CAD build for the part. Positions are in the model's coordinates, mm. A direction names the side the tool comes from. Round coordinates to 2 decimals unless told otherwise and drop trailing zeros. Order: outer loops, then holes, each group sorted by start corner. A loop starts at its lowest first (then second) coordinate and runs counter-clockwise, first axis right, second up. Notation, with made-up numbers: M 14,58.5 L 40,58.5 A28 cw 40,97.5 Z; hole C 40.25,-35 d1. An arc over 180 degrees is marked long. Answer as CSV lines item,"result". Start each with the question number.
```python
from build123d import *

# Parameters (mm, degrees)
SKETCH2_W           = 15
SKETCH2_H           = 15
SKETCH2_W_2         = 30
SKETCH2_R           = 4.15
BOSS_EXTRUDE1_DEPTH = 10
SKETCH2_3_W         = 15
SKETCH2_3_H         = 15
SKETCH2_3_W_2       = 30
SKETCH2_3_R         = 4.15
BOSS_EXTRUDE2_DEPTH = 10
SKETCH4_R           = 1.6
CUT_EXTRUDE1_DEPTH  = 36
CUT_EXTRUDE2_START  = -6.25
SKETCH4_3_R         = 1.6
CUT_EXTRUDE2_DEPTH  = 2.5
SKETCH5_W           = 45
SKETCH5_H           = 5
BOSS_EXTRUDE3_DEPTH = 75
SKETCH6_W           = 45
SKETCH6_H           = 5
BOSS_EXTRUDE4_DEPTH = 15
SKETCH7_W           = 5
SKETCH7_H           = 20
BOSS_EXTRUDE5_DEPTH = 45
CUT_EXTRUDE3_REACH  = 119.58
SKETCH8_R           = 1.6
CUT_EXTRUDE4_START  = -1.25
CUT_EXTRUDE4_DEPTH  = 2.5


with BuildPart() as part:
    # Sketch2 → Boss-Extrude1 (new body)
    with BuildSketch(Plane(origin=(0, 0, 0), x_dir=(1, 0, 0), z_dir=(0, 1, 0))):
        with Locations((22.5, 0)):
            Rectangle(SKETCH2_W, SKETCH2_H)
        Rectangle(SKETCH2_W_2, SKETCH2_H)
        with Locations(Location((7.5, 0, 0), (0, 0, 270))):
            Circle(SKETCH2_R, mode=Mode.SUBTRACT)
        with Locations(Location((-7.5, 0, 0), (0, 0, 270))):
            Circle(SKETCH2_R, mode=Mode.SUBTRACT)
    extrude(amount=BOSS_EXTRUDE1_DEPTH)

    # Sketch2_3 → Boss-Extrude2 (add)
    with BuildSketch(Plane(origin=(0, 0, 0), x_dir=(1, 0, 0), z_dir=(0, 1, 0))):
        with Locations((22.5, 0)):
            Rectangle(SKETCH2_3_W, SKETCH2_3_H)
        Rectangle(SKETCH2_3_W_2, SKETCH2_3_H)
        with Locations(Location((7.5, 0, 0), (0, 0, 270))):
            Circle(SKETCH2_3_R, mode=Mode.SUBTRACT)
        with Locations(Location((-7.5, 0, 0), (0, 0, 270))):
            Circle(SKETCH2_3_R, mode=Mode.SUBTRACT)
        with Locations(Location((-7.5, 0, 0), (0, 0, 270))):
            Circle(SKETCH2_3_R)
        with Locations(Location((7.5, 0, 0), (0, 0, 270))):
            Circle(SKETCH2_3_R)
    extrude(amount=-BOSS_EXTRUDE2_DEPTH)

    # Sketch4 → Cut-Extrude1 (cut, through all)
    with BuildSketch(Plane.XY.offset(7.5)):
        with Locations((22.5, 5)):
            Circle(SKETCH4_R)
        with Locations((22.5, -5)):
            Circle(SKETCH4_R)
    extrude(amount=-CUT_EXTRUDE1_DEPTH, mode=Mode.SUBTRACT)

    # Sketch4_3 → Cut-Extrude2 (cut)
    with BuildSketch(Plane.XY.offset(7.5).offset(CUT_EXTRUDE2_START)):
        Polygon((22.5, 8.435234102), (19.525, 6.717617051), (19.525, 3.282382949), (22.5, 1.564765898), (25.475, 3.282382949), (25.475, 6.717617051), align=None)
        with Locations((22.5, 5)):
            Circle(SKETCH4_3_R, mode=Mode.SUBTRACT)
        Polygon((22.5, -8.435234102), (25.475, -6.717617051), (25.475, -3.282382949), (22.5, -1.564765898), (19.525, -3.282382949), (19.525, -6.717617051), align=None)
        with Locations((22.5, -5)):
            Circle(SKETCH4_3_R, mode=Mode.SUBTRACT)
    extrude(amount=-CUT_EXTRUDE2_DEPTH, mode=Mode.SUBTRACT)

    # Sketch5 → Boss-Extrude3 (add)
    with BuildSketch(Plane.XY.offset(7.5)):
        with Locations((7.5, -7.5)):
            Rectangle(SKETCH5_W, SKETCH5_H)
    extrude(amount=BOSS_EXTRUDE3_DEPTH)

    # Sketch6 → Boss-Extrude4 (add)
    with BuildSketch(Plane(origin=(0, -5, 0), x_dir=(1, 0, 0), z_dir=(0, 1, 0))):
        with Locations((7.5, -80)):
            Rectangle(SKETCH6_W, SKETCH6_H)
    extrude(amount=BOSS_EXTRUDE4_DEPTH)

    # Sketch7 → Boss-Extrude5 (add)
    with BuildSketch(Plane(origin=(30, 0, 0), x_dir=(0, 0, -1), z_dir=(1, 0, 0))):
        with Locations((-80, 0)):
            Rectangle(SKETCH7_W, SKETCH7_H)
    extrude(amount=BOSS_EXTRUDE5_DEPTH)

    # Sketch8 → Cut-Extrude3 (cut, up to next)
    with BuildSketch(Plane.XY.offset(82.5), mode=Mode.PRIVATE) as cut_extrude3_sk1:
        with Locations((5, 3.75)):
            Circle(SKETCH8_R)
    cut_extrude3_tool1 = extrude(cut_extrude3_sk1.sketch, amount=-CUT_EXTRUDE3_REACH, mode=Mode.PRIVATE) & part.part
    # Sketch8 → Cut-Extrude3 (cut, up to next)
    with BuildSketch(Plane.XY.offset(82.5), mode=Mode.PRIVATE) as cut_extrude3_sk2:
        with Locations((40, 3.75)):
            Circle(SKETCH8_R)
    cut_extrude3_tool2 = extrude(cut_extrude3_sk2.sketch, amount=-CUT_EXTRUDE3_REACH, mode=Mode.PRIVATE) & part.part
    add(cut_extrude3_tool1.solids().sort_by_distance((5, 3.75, 82.5))[0], mode=Mode.SUBTRACT)
    add(cut_extrude3_tool2.solids().sort_by_distance((40, 3.75, 82.5))[0], mode=Mode.SUBTRACT)

    # Sketch9 → Cut-Extrude4 (cut)
    with BuildSketch(Plane.XY.offset(82.5).offset(CUT_EXTRUDE4_START)):
        Polygon((5, 0.314765898), (7.975, 2.032382949), (7.975, 5.467617051), (5, 7.185234102), (2.025, 5.467617051), (2.025, 2.032382949), align=None)
        Polygon((40, 0.314765898), (42.975, 2.032382949), (42.975, 5.467617051), (40, 7.185234102), (37.025, 5.467617051), (37.025, 2.032382949), align=None)
    extrude(amount=-CUT_EXTRUDE4_DEPTH, mode=Mode.SUBTRACT)


solid = part.part
```
Q1. Tool access for faces 1 (the flat face through (2.025, 4, 80)), 2 (the cylindrical face through (-4.695, 4.93, -3.059)), 3 (the cylindrical face through (4.65, 2.19, 78.13)): list every direction of +Z, -Z, +X, -X, +Y, -Y with a clear straight run to the whole face (end or side of a thin tool).
Q2. Drop flat-ended pins along their axis: P1, Ø5, axis at x = 40, y = 3.5, coming from the -Z side; P2, Ø12, axis at x = 35, z = 31, coming from the +Y side; P3, Ø3, axis at x = 22.5, y = -5, coming from the -Z side. Give the stop position or say it passes through.
Q3. Band-saw the part on B-B, the plane z = 0. Write the cut outline in (x, y) (3 decimals), then the cut area to 3 significant figures.
Q4. Mould opens along Z. For faces 4 (the flat face through (7, -5, 42)), 5 (the cylindrical face through (24.026, -4.519, 4.419)), 6 (the flat face through (29, 0, 77.5)) say: +Z half, -Z half, draft (parallel to the pull), parting line (faces both ways), or undercut.
Q5. Band-saw the part on C-C, the plane z = 70.5. Write the cut outline in (x, y), then the cut area to 3 significant figures.
Q6. Probe line 1 along Z through (x, y) = (24, -4); line 2 along X through (y, z) = (5, 0) (3 decimals); line 3 along Z through (x, y) = (5.5, -3). List the from-to ranges inside material, lowest first. Write a range as from..to.
Q7. Band-saw the part on D-D, the plane x = 61. Write the cut outline in (y, z), then the cut area to 3 significant figures.
Q8. Band-saw the part on A-A, the plane x = -7.5. Write the cut outline in (y, z).
Answer:
1,face 1,"none"
1,face 2,"+Y"
1,face 3,"+Z"
2,P1,"stops at z = 77.5"
2,P2,"stops at y = -5"
2,P3,"stops at z = 7.5"
3,outline,"M -15,-10 L 30,-10 L 30,10 L 11.65,10 L 11.65,0 L 3.35,0 L 3.35,10 L -3.35,10 L -3.35,0 L -11.65,0 L -11.65,10 L -15,10 Z; hole M 19.525,-6.718 L 22.5,-8.435 L 25.475,-6.718 L 25.475,-3.282 L 22.5,-1.565 L 19.525,-3.282 Z; hole M 19.525,3.282 L 22.5,1.565 L 25.475,3.282 L 25.475,6.718 L 22.5,8.435 L 19.525,6.718 Z"
3,area,"673 mm^2"
4,face 4,"undercut"
4,face 5,"draft"
4,face 6,"undercut"
5,outline,"M -15,-10 L 30,-10 L 30,-5 L -15,-5 Z"
5,area,"225 mm^2"
6,line 1,"z = -7.5..-1.25, 1.25..7.5, 77.5..82.5"
6,line 2,"x = -15..-11.65, -3.35..3.35, 11.65..19.525, 25.475..30"
6,line 3,"z = -7.5..7.5, 77.5..82.5"
7,outline,"M -10,77.5 L 10,77.5 L 10,82.5 L -10,82.5 Z"
7,area,"100 mm^2"
8,outline,"M -10,-7.5 L 10,-7.5 L 10,-4.15 L 0,-4.15 L 0,4.15 L 10,4.15 L 10,7.5 L -5,7.5 L -5,77.5 L 10,77.5 L 10,82.5 L -10,82.5 Z"
